Verification items for the finished model (mm, model axes). Face numbers are marked on the shaded views. A direction names the side the tool comes from. Coordinates: 2 decimals unless noted, no trailing zeros. Loops run counter-clockwise (first coordinate to the right, second up) from the corner with the lowest first, then second, coordinate; pieces in that order, holes last. Notation, with made-up numbers: (-7.5, 38.25) - (29.5, 38.25) arc R3 cw to (29.5, 43.25) - close; hole circle Ø10 at (-17, -34.75). An arc over 180 degrees is marked (long way). Answer as CSV lines item,"result". Start each with the question number.
1. Cross-section at C-C (z = -20). Enter the section's corners in (x, y).
2. Cross-section at D-D (y = 30). Enter the section's corners in (x, z), plus the area to 3 significant figures.
3. Material ranges on line 1 (X direction, y = 63.5, z = -26); line 2 (Y direction, x = -71, z = -54.5); line 3 (Z direction, x = -42.5, y = 48), recorded low to high. Write a range as [from, to].
4. Cross-section at A-A (x = -62). Enter the section's corners in (y, z).
5. Release check for a two-part mould opening along Y. For the marked faces 6, 7 and 8 record: pulls with the +Y half, pulls with the -Y half, needs draft (parallel to the pull), parting line crosses it, or undercut.
6. Gauge pin test, flat ends, axial feed: P1, Ø3, axis at x = -32.5, y = 42.5, coming from the +Z side; P2, Ø25, axis at y = 21, z = -16, coming from the +X side; P3, Ø18.5, axis at x = -75, y = 35.5, coming from the -Z side; P4, Ø1, axis at x = -42, y = 69.5, coming from the -Z side. Record the tip position at first contact, or that the pin passes through.
7. Set-up check for the marked faces 1, 2, 3, 4 and 5: record each of +Z, -Z, +X, -X, +Y, -Y from which the full face is reachable in a straight line by a thin tool's end or side.
8. Cross-section at B-B (y = 47). Enter the section's corners in (x, z).
Autodesk Inventor part; units mm, degrees
ref_plane "YZ Plane" through (0, 0, 0) normal (1, 0, 0) x (0, 1, 0)
ref_plane "XZ Plane" through (0, 0, 0) normal (0, 1, 0) x (-1, 0, 0)
ref_plane "XY Plane" through (0, 0, 0) normal (0, 0, 1) x (1, 0, 0)
sketch "Esboço1" plane through (0, 0, 0) normal (0, 1, 0) x (-1, 0, 0)
  line L0 (0, 0) -> (100, 0)
  line L1 (100, 0) -> (100, -100)
  line L2 (100, -100) -> (0, -100)
  line L3 (0, -100) -> (0, 0)
  dimension "d0" = 100
  dimension "d1" = 100
extrude "Extrusão1" add sketch "Esboço1" along normal blind 85
sketch "Esboço2" plane through (0, 0, 0) normal (1, 0, 0) x (0, 0, -1)
  line L0 (100, 0) -> (0, 0)
  line L1 (0, 0) -> (20, 0)
  circle A0 centre (20, 15) radius 15
  line L2 (35, 15) -> (35, 0)
  line L3 (5, 15) -> (5, 0)
  line L4 (100, 85) -> (0, 85)
  line L5 (100, 0) -> (100, 85)
  line L6 (0, 85) -> (25, 85)
  line L7 (100, 10) -> (100, 0)
  line L8 (100, 0) -> (95, 0)
  line L9 (0, 0) -> (0, 85)
  line L10 (100, 0) -> (89.5, 0)
  line L11 (82.5, 12.5) -> (82.5, 49.1652)
  line L12 (0, 85) -> (55, 85)
  line L13 (100, 85) -> (100, 0)
  line L14 (100, 0) -> (0, 0)
  line L15 (0, 0) -> (0, 85)
  line L16 (78.5573, 59.3011) -> (55, 85)
  arc A1 (82.5, 49.1652) -> (78.5573, 59.3011) centre (67.5, 49.1652) ccw
  arc A2 (82.5, 12.5) -> (95, 0) centre (95, 12.5) ccw
  point P0 (82.5, 0)
  point P1 (82.5, 85)
  point P2 (5, 0)
  dimension "d6" = 30
  dimension "d8" = 17.5
  dimension "d11" = 15
  dimension "d12" = 12.5
extrude "Extrusão2" cut sketch "Esboço2" against normal blind 100 contours L0 A2 L11 A1 L16 L4 L5
extrude "Extrusão3" cut sketch "Esboço2" against normal blind 45 contours L0 A0 L2 | L0 L3 A0 | A0
sketch "Esboço3" plane through (-100, 0, 0) normal (-1, 0, 0) x (0, 0, 1)
  arc A0 (-5, 15) -> (-35, 15) centre (-20, 15) ccw
  line L0 (-20, 15) -> (-20, 0)
  line L1 (-95, 0) -> (0, 0)
  circle A1 centre (-20, 15) radius 15
  line L2 (-35, 15) -> (-35, -0.9881)
  line L3 (-5, 0) -> (-5, 15)
  line L4 (-5, 15) -> (-5, 0)
  line L5 (-35, 0) -> (-5, 0)
extrude "Extrusão4" cut sketch "Esboço3" against normal blind 45
sketch "Esboço4" plane through (-100, 0, 0) normal (0, 0, 1) x (1, 0, 0)
  line L0 (0, 0) -> (0, 12.5)
  line L1 (0, 12.5) -> (0, 17.5)
  line L2 (0, 49.1652) -> (0, 12.5)
  line L3 (0, 17.5) -> (0, 7.5)
  line L4 (0, 17.5) -> (40, 17.5)
  line L5 (45, 15) -> (45, 30)
  line L6 (40, 17.5) -> (40, 7.5)
  line L7 (40, 7.5) -> (0, 7.5)
  line L8 (100, 12.5) -> (100, 49.1652)
  line L9 (100, 17.5) -> (100, 7.5)
  line L10 (100, 7.5) -> (60, 7.5)
  line L11 (60, 7.5) -> (60, 17.5)
  line L12 (60, 17.5) -> (100, 17.5)
  line L13 (45, 30) -> (45, 34)
  line L14 (45, 34) -> (95, 34)
  line L15 (45, 34) -> (5, 34)
  line L16 (5, 34) -> (95, 34)
  line L17 (5, 34) -> (5, 82.5)
  line L18 (5, 82.5) -> (95, 82.5)
  line L19 (95, 82.5) -> (95, 34)
  line L20 (5, 34) -> (5, 61.5)
  line L21 (5, 34) -> (5, 58.25)
  line L22 (5, 58.25) -> (95, 58.25)
  line L23 (95, 58.25) -> (95, 34)
  line L24 (95, 34) -> (5, 34)
  point P0 (100, 0)
  dimension "d20" = 10
  dimension "d22" = 40
  dimension "d27" = 48.5
extrude "Extrusão5" cut sketch "Esboço4" against normal blind 10 contours L0 L1 L4 L6 L7 | L9 L10 L11 L12 L8
extrude "Extrusão6" cut sketch "Esboço4" against normal blind 52 contours L22 L17 L18 L19
extrude "Extrusão7" cut sketch "Esboço4" against normal blind 60 contours L15 L17 L22 L19 L14
sketch "Esboço5" plane through (0, 85, 0) normal (0, 1, 0) x (1, 0, 0)
  line L0 (-95, 0) -> (-95, 52)
  line L1 (-95, 4.5451) -> (-95, 52)
  line L2 (-5, 0) -> (-5, 52)
  line L3 (-95, 52) -> (-5, 52)
  line L4 (-5, 52) -> (-5, 4.5451)
  line L5 (-5, 4.5451) -> (-95, 4.5451)
  point P0 (0, 0)
extrude "Extrusão8" cut sketch "Esboço5" against normal blind 10.75
sketch "Esboço6" plane through (-100, 12.5, -82.5) normal (-1, 0, 0) x (0, 0, 1)
  arc A0 (77.2902, 5) -> (47.5, 2.5) centre (62.5, 2.5) ccw
  circle A1 centre (62.5, 2.5) radius 16.5
  line L0 (46, 2.5) -> (46, -12.5)
  line L1 (79, 2.5) -> (79, -12.5)
  line L2 (82.5, 5) -> (82.5, -5)
  line L3 (46, -12.5) -> (79, -12.5)
  line L4 (77.5, -12.5) -> (82.5, -12.5)
  dimension "d37" = 33
extrude "Extrusão9" cut sketch "Esboço6" against normal blind 45 contours A1 L3 | L1 L3 A1 | A1 L3 L0 picked at (60.7652, -1.3921)
sketch "Esboço7" plane through (0, 12.5, -82.5) normal (1, 0, 0) x (0, 0, -1)
  arc A0 (-46, 2.5) -> (-79, 2.5) centre (-62.5, 2.5) ccw
  circle A1 centre (-62.5, 2.5) radius 16.5
  line L0 (-79, -12.5) -> (-82.5, -12.5)
  line L1 (-79, 2.5) -> (-79, -12.5)
  line L2 (-79, -12.5) -> (-46, -12.5)
  line L3 (-46, -12.5) -> (-46, 2.5)
  dimension "d40" = 33
extrude "Extrusão10" cut sketch "Esboço7" against normal blind 45 contours A1 L2 A0 | L3 L2 A1 | A1 L2 L1
properties part number "mini sumô rascunho v2"
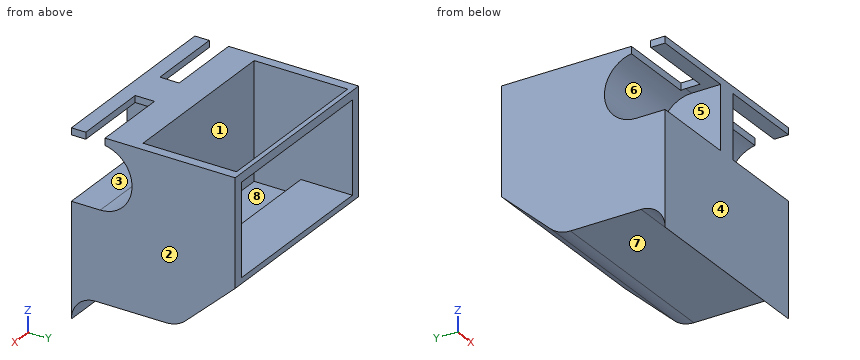
Values follow:
1,outline,"(-100, 31.5) - (-55, 31.5) - (-55, 0) - (-45, 0) - (-45, 31.5) - (0, 31.5) - (0, 85) - (-5, 85) - (-5, 34) - (-95, 34) - (-95, 85) - (-100, 85) - close"
2,outline,"(-100, -82.5) - (0, -82.5) - (0, -26.87) - (-45, -26.87) - (-45, -13.13) - (0, -13.13) - (0, 0) - (-100, 0) - (-100, -13.13) - (-55, -13.13) - (-55, -26.87) - (-100, -26.87) - close"
2,area,"7,010 mm²"
3,line 1,"x = [-100, -95], [-5, 0]"
3,line 2,"y = [0, 34], [58.25, 85]"
3,line 3,"z = [-82.5, -60]"
4,outline,"(0, -95) arc R12.5 cw to (12.5, -82.5) - (49.17, -82.5) arc R15 ccw to (59.3, -78.56) - (85, -55) - (85, -52) - (58.25, -52) - (58.25, -60) - (34, -60) - (34, 0) - (17.5, 0) - (17.5, -3.69) arc R16.5 cw to (15, -36.5) - (0, -36.5) - close; (0, -3.5) - (7.5, -3.5) - (7.5, 0) - (0, 0) - close; (82.5, -4.55) - (85, -4.55) - (85, 0) - (82.5, 0) - close"
5,face 6,"pulls with the -Y half"
5,face 7,"needs draft"
5,face 8,"undercut"
6,P1,"stops at z = -60"
6,P2,"stops at x = 0"
6,P3,"stops at z = -82.5"
6,P4,"stops at z = -69.67"
7,face 1,"+Z"
7,face 2,"+Z, -Z, +X, +Y, -Y"
7,face 3,"+X, -Y"
7,face 4,"+Z, -Z, +X, -X, -Y"
7,face 5,"-X, -Y"
8,outline,"(-100, -82.5) - (0, -82.5) - (0, 0) - (-5, 0) - (-5, -60) - (-95, -60) - (-95, 0) - (-100, 0) - close"
